Check sheet for the modelled part. Datum: model origin and axes. Units: mm. A direction names the side the tool comes from. Coordinates: 2 decimals unless noted, no trailing zeros. Write each loop counter-clockwise with the first axis right and the second up, starting at its lowest first coordinate (ties: lowest second). Pieces come first, ordered by that corner, then holes. Notation, with made-up numbers: M -20,6.5 L 32,6.5 A12 ccw 32,19.5 Z; hole C -35.75,9.25 d7. An arc over 180 degrees is marked long. Answer as CSV lines item,"result".
from build123d import *

# Parameters (mm, degrees)
CROQUIS1_W              = 90
CROQUIS1_H              = 200
SALIENTE_EXTRUIR1_DEPTH = 5
CROQUIS2_W              = 90
CROQUIS2_H              = 5
SALIENTE_EXTRUIR2_DEPTH = 64
CROQUIS3_W              = 36
CROQUIS3_H              = 42
SALIENTE_EXTRUIR3_DEPTH = 1
CROQUIS4_R              = 3
CORTAR_EXTRUIR1_DEPTH   = 201
CROQUIS5_W              = 27
CROQUIS5_H              = 190
CORTAR_EXTRUIR3_DEPTH   = 6
CROQUIS6_W              = 27
CROQUIS6_H              = 52
CORTAR_EXTRUIR4_DEPTH   = 201


with BuildPart() as part:
    # Croquis1 → Saliente-Extruir1 (new body)
    with BuildSketch(Plane.XY):
        Rectangle(CROQUIS1_W, CROQUIS1_H)
    extrude(amount=-SALIENTE_EXTRUIR1_DEPTH)

    # Croquis2 → Saliente-Extruir2 (add)
    with BuildSketch(Plane.XY):
        with Locations((0, 97.5)):
            Rectangle(CROQUIS2_W, CROQUIS2_H)
        with Locations((0, -97.5)):
            Rectangle(CROQUIS2_W, CROQUIS2_H)
    extrude(amount=SALIENTE_EXTRUIR2_DEPTH)

    # Croquis3 → Saliente-Extruir3 (add)
    with BuildSketch(Plane.XY):
        with Locations((0, 35)):
            Rectangle(CROQUIS3_W, CROQUIS3_H)
        with Locations((0, -35)):
            Rectangle(CROQUIS3_W, CROQUIS3_H)
    extrude(amount=SALIENTE_EXTRUIR3_DEPTH)

    # Croquis4 → Cortar-Extruir1 (cut, through all)
    with BuildSketch(Plane(origin=(0, 100, 0), x_dir=(1, 0, 0), z_dir=(0, 1, 0))):
        with Locations((-25, -55.5)):
            Circle(CROQUIS4_R)
        with Locations((0, -55.5)):
            Circle(CROQUIS4_R)
        with Locations((25, -55.5)):
            Circle(CROQUIS4_R)
    extrude(amount=-CORTAR_EXTRUIR1_DEPTH, mode=Mode.SUBTRACT)

    # Croquis5 → Cortar-Extruir3 (cut, through all)
    with BuildSketch(Plane.XY):
        with Locations((-31.5, 0)):
            Rectangle(CROQUIS5_W, CROQUIS5_H)
        with Locations((31.5, 0)):
            Rectangle(CROQUIS5_W, CROQUIS5_H)
    extrude(amount=-CORTAR_EXTRUIR3_DEPTH, mode=Mode.SUBTRACT)

    # Croquis6 → Cortar-Extruir4 (cut, through all)
    with BuildSketch(Plane(origin=(0, 100, 0), x_dir=(1, 0, 0), z_dir=(0, 1, 0))):
        with Locations((-31.5, -21)):
            Rectangle(CROQUIS6_W, CROQUIS6_H)
        with Locations((31.5, -21)):
            Rectangle(CROQUIS6_W, CROQUIS6_H)
    extrude(amount=-CORTAR_EXTRUIR4_DEPTH, mode=Mode.SUBTRACT)


solid = part.part
1) Section check B-B, the plane z = 21. Record the boundary of the cut face in (x, y).
Answer key:
outline,"M -18,-100 L 18,-100 L 18,-95 L -18,-95 Z; M -18,95 L 18,95 L 18,100 L -18,100 Z"
2) Tool access check on faces 1 (the face through (-1, 100, 37)), 2 (the face through (31, -97, 47)), 3 (the face through (24.609, -97.465, 52.526)), 4 (the face through (0, 76, 0)), 5 (the face through (-32, -97, 47)). Record the directions out of +Z, -Z, +X, -X, +Y, -Y that give a thin tool (end or side, any length) a straight path to the whole face; none if there is none.
Answer key:
face 1,"+Z, -Z, +X, -X, +Y"
face 2,"-Z, +X, +Y, -Y"
face 3,"+Y, -Y"
face 4,"+Z, +X, -X"
face 5,"-Z, -X, +Y, -Y"
3) Section check A-A, the plane x = 25. Record the boundary of the cut face in (y, z).
Answer key:
outline,"M -100,47 L -95,47 L -95,52.5 L -100,52.5 Z; M -100,58.5 L -95,58.5 L -95,64 L -100,64 Z; M 95,47 L 100,47 L 100,52.5 L 95,52.5 Z; M 95,58.5 L 100,58.5 L 100,64 L 95,64 Z"
4) Section check C-C, the plane z = 55.5. Give the number of separate pieces and of enclosed holes in the cut face, plus the area to 3 significant figures.
Answer key:
separate pieces,"8"
enclosed holes,"0"
area,"720 mm2"
5) Section check D-D, the plane x = -11.5. Record the boundary of the cut face in (y, z), plus the area to 3 significant figures.
Answer key:
outline,"M -100,-5 L 100,-5 L 100,64 L 95,64 L 95,0 L 56,0 L 56,1 L 14,1 L 14,0 L -14,0 L -14,1 L -56,1 L -56,0 L -95,0 L -95,64 L -100,64 Z"
area,"1,720 mm2"
6) Mould release check, pull along X, two halves, no side actions. Record for faces 6 (the face through (-25.391, 97.535, 52.526)), 7 (the face through (18, 0, -4)), 8 (the face through (-1, -100, 38)), 9 (the face through (-0.391, -97.465, 52.526)): pulls with the +X half, pulls with the -X half, needs draft (parallel to the pull), parting line crosses it, or undercut.
Answer key:
face 6,"undercut"
face 7,"pulls with the +X half"
face 8,"needs draft"
face 9,"undercut"
7) Thickness scan on line 1 along X through (y, z) = (-97, 55); line 2 along Z through (x, y) = (25, -96); line 3 along Y through (x, z) = (-10, 47). Record the ranges inside material, lowest first.
Answer key:
line 1,"x = -45 to -27.96, -22.04 to -2.96, 2.96 to 22.04, 27.96 to 45"
line 2,"z = 47 to 52.5, 58.5 to 64"
line 3,"y = -100 to -95, 95 to 100"
8) Depth check by flat-ended pin: P1, Ø22.5, axis at x = 5.5, y = 3, coming from the +Z side; P2, Ø10, axis at x = 26, z = 26.5, coming from the +Y side; P3, Ø5.5, axis at x = -31.5, y = 97.5, coming from the -Z side; P4, Ø8, axis at x = -6.5, y = -70, coming from the +Z side. Enter the tip coordinate at first touch or a pass-through.
Answer key:
P1,"stops at z = 1"
P2,"passes through"
P3,"stops at z = 47"
P4,"stops at z = 0"
